Build history of the part. All positions in model axes, mm. Give positions to 0.01 mm unless a question says otherwise; leave off trailing zeros. Order: outer loops, then holes, each group sorted by start corner. A loop starts at its lowest first (then second) coordinate and runs counter-clockwise, first axis right, second up. Notation, with made-up numbers: (62.5, 36.5) -> (101.5, 36.5) arc R17 ccw to (101.5, 69.5) -> close; hole circle Ø10 at (10, 61.25). An arc over 180 degrees is marked (long way). Write item = value, one per line. Start each with the question number.
Autodesk Inventor part; units mm, degrees
ref_plane "YZ Plane" through (0, 0, 0) normal (1, 0, 0) x (0, 1, 0)
ref_plane "XZ Plane" through (0, 0, 0) normal (0, 1, 0) x (-1, 0, 0)
ref_plane "XY Plane" through (0, 0, 0) normal (0, 0, 1) x (1, 0, 0)
ref_plane "Work Plane1" through (18.544, -14.9845, 0) normal (0, 0, 1) x (1, 0, 0)
sketch "Sketch1" plane through (18.544, -14.9845, 0) normal (0, 0, 1) x (1, 0, 0)
  line L0 (-31.544, 764.9845) -> (-24.544, 764.9845)
  line L1 (-24.544, 764.9845) -> (-24.544, 1014.9845)
  line L2 (-31.544, 1014.9845) -> (-24.544, 1014.9845)
  line L3 (-31.544, 764.9845) -> (-31.544, 1014.9845)
  line L4 (-18.544, 764.9845) -> (-11.544, 764.9845)
  line L5 (-11.544, 764.9845) -> (-11.544, 1014.9845)
  line L6 (-18.544, 1014.9845) -> (-11.544, 1014.9845)
  line L7 (-18.544, 764.9845) -> (-18.544, 1014.9845)
  circle A0 centre (-21.544, 754.9845) radius 2.5
  line L8 (-21.544, 754.9845) -> (-21.544, 786.7892) construction
  line L9 (-31.544, 764.9845) -> (-27.7385, 753.0151)
  line L10 (-15.3496, 753.0151) -> (-11.544, 764.9845)
  circle A1 centre (-21.544, 754.9845) radius 6.5
  line L11 (-31.544, 764.9845) -> (-31.544, 786.9845)
  line L12 (-31.544, 786.9845) -> (-11.544, 786.9845)
  line L13 (-11.544, 764.9845) -> (-11.544, 786.9845)
  point P0 (-18.544, 14.9845)
  point P1 (-21.544, 769.9845)
  point P2 (-21.544, 781.9845)
  dimension "d0" = 5
  dimension "d1" = 12
  dimension "d2" = 4
  dimension "d3" = 5
extrude "Extrusion1" add sketch "Sketch1" along normal blind 4 contours L3 L12 L1 L0 | L0 L1 L12 L7 L4 L10 A1 L9 | A1 | L12 L5 L4 L7 | A0
sketch "Sketch2" plane through (18.544, -14.9845, 4) normal (0, 0, 1) x (1, 0, 0)
  point P0 (-18.544, 14.9845)
  point P1 (-21.544, 769.9845)
  point P2 (-21.544, 781.9845)
  point P3 (-21.544, 754.9845)
hole "Hole1" at (-3, 755, 4) at (-3, 767, 4) direction (0, 0, -1) diameter 4.5 end through all countersink diameter 8.6 countersink angle 90
hole "Hole2" at (-3, 740, 4) direction (0, 0, -1) diameter 5.5 end through all countersink diameter 10.4 countersink angle 90
properties part number "belt_tentioner_plane"
(1) Cut at D-D, the plane y = 740. Give the cut face in (x, z).
(2) Wall check: line 1 (Y direction, x = -3, z = 1.2); line 2 (Y direction, x = -2, z = 2.65); line 3 (X direction, y = 755, z = 1.5). Give the ranges that are in metal, low to high. Write a range as [from, to].
(3) Cut at C-C, the plane z = 0.8. Give the cut face in (x, y).
(4) Cut at A-A, the plane x = -3. Give the cut face in (y, z).
(5) Cut at B-B, the plane y = 755. Give the cut face in (x, z).
(6) Mould opens along X. For faces 1 (the face through (-2.9, 769.4, 2.1)), 2 (the face through (-13, 761, 2)), 3 (the face through (-2.9, 733.5, 2)) say: released by +X, released by -X, zero draft, split by the parting line, or undercut.
(7) Flat gauge pins, fed straight in: P1, Ø7, axis at x = -3, y = 740, coming from the +Z side; P2, Ø2, axis at x = -6.5, z = 2, coming from the -Y side. Where does each tip first touch, or does it go through?
Results:
q1.outline = (-9.82, 0) -> (-5.75, 0) -> (-5.75, 1.55) -> (-8.2, 4) -> (-9.82, 4) -> close; (-0.25, 0) -> (3.82, 0) -> (3.82, 4) -> (2.2, 4) -> (-0.25, 1.55) -> close
q2.line_1 = [733.5, 737.25], [742.75, 752.75], [757.25, 764.75], [769.25, 772]
q2.line_2 = [733.58, 736.28], [743.72, 752.22], [757.78, 764.22], [769.78, 772]
q2.line_3 = [-13, -5.25], [-0.75, 7]
q3.outline = (-13, 750) -> (-9.19, 738.03) arc R6.5 ccw to (3.19, 738.03) -> (7, 750) -> (7, 772) -> (-13, 772) -> close; hole circle Ø5.5 at (-3, 740); hole circle Ø4.5 at (-3, 755); hole circle Ø4.5 at (-3, 767)
q4.outline = (733.5, 0) -> (737.25, 0) -> (737.25, 1.55) -> (734.8, 4) -> (733.5, 4) -> close; (742.75, 0) -> (752.75, 0) -> (752.75, 1.95) -> (750.7, 4) -> (745.2, 4) -> (742.75, 1.55) -> close; (757.25, 0) -> (764.75, 0) -> (764.75, 1.95) -> (762.7, 4) -> (759.3, 4) -> (757.25, 1.95) -> close; (769.25, 0) -> (772, 0) -> (772, 4) -> (771.3, 4) -> (769.25, 1.95) -> close
q5.outline = (-13, 0) -> (-5.25, 0) -> (-5.25, 1.95) -> (-7.3, 4) -> (-13, 4) -> close; (-0.75, 0) -> (7, 0) -> (7, 4) -> (1.3, 4) -> (-0.75, 1.95) -> close
q6.face_1 = undercut
q6.face_2 = released by -X
q6.face_3 = split by the parting line
q7.P1 = 2.3
q7.P2 = 734
